Source: CAD feature listing. Evaluate the final solid. Frame: model axes, mm. Face numbers are marked on the shaded views. A direction names the side the tool comes from. Coordinates: 2 decimals unless noted, no trailing zeros. Loops run counter-clockwise (first coordinate to the right, second up) from the corner with the lowest first, then second, coordinate; pieces in that order, holes last. Notation, with made-up numbers: (-6.75, -27.75) - (21.25, -27.75) arc R21 ccw to (21.25, 1.25) - close; hole circle Ø9 at (64.5, 55). An arc over 180 degrees is marked (long way). Use CSV: the item, a comma, the result in double quotes. Start each with the question number.
```python
from build123d import *

# Parameters (mm, degrees)
BOSS_EXTRUDE1_DEPTH      = 28.22702
BOSS_EXTRUDE1_DEPTH_BACK = 27.08402
SKETCH2_R                = 40.9575
CUT_EXTRUDE1_DEPTH       = 152.701320166
CUT_EXTRUDE2_DEPTH       = 152.701320166


with BuildPart() as part:
    # Sketch1 → Boss-Extrude1 (new, two sides: drawn at the far end of the back side and taken through both)
    with BuildSketch(Plane(origin=(0, 0, 0), x_dir=(1, 0, 0), z_dir=(0, 1, 0)).offset(-BOSS_EXTRUDE1_DEPTH_BACK)):
        with BuildLine():
            Line((-35.721676258, -109.931199839), (-58.1025, -56.069211009))
            Line((-58.1025, -56.069211009), (-58.1025, -54.569599156))
            Line((-58.1025, -54.569599156), (-58.1025, 64.002262273))
            Line((-58.1025, 64.002262273), (-46.861446545, 91.314524953))
            ThreePointArc((-46.861446545, 91.314524953), (-41.24957855, 98.176226775), (-32.76841286, 100.75418))
            Line((-32.76841286, 100.75418), (30.359183597, 100.75418))
            ThreePointArc((30.359183597, 100.75418), (40.293026824, 97.071703902), (45.426195478, 87.803885872))
            Line((45.426195478, 87.803885872), (49.528165732, 60.811582924))
            ThreePointArc((49.528165732, 60.811582924), (51.439588659, 56.249062009), (55.27903878, 53.129966389))
            Line((55.27903878, 53.129966389), (78.152801145, 42.463755827))
            ThreePointArc((78.152801145, 42.463755827), (80.557519892, 40.354874086), (81.452537779, 37.284206824))
            Line((81.452537779, 37.284206824), (81.452537779, 31.863274858))
            ThreePointArc((81.452537779, 31.863274858), (80.517086587, 28.730043586), (78.016968856, 26.622528826))
            Line((78.016968856, 26.622528826), (63.334487079, 20.236471377))
            ThreePointArc((63.334487079, 20.236471377), (58.494345864, 15.83382392), (57.342134405, 9.393118961))
            Line((57.342134405, 9.393118961), (57.442982796, 8.729503635))
            ThreePointArc((57.442982796, 8.729503635), (57.930235286, 4.470832805), (58.1021964, 0.187828999))
            ThreePointArc((58.1021964, 0.187828999), (59.236377824, -4.444212154), (62.359072928, -8.048507927))
            Line((62.359072928, -8.048507927), (79.05801487, -19.969280438))
            ThreePointArc((79.05801487, -19.969280438), (80.818765563, -22.004906493), (81.452537779, -24.620694942))
            Line((81.452537779, -24.620694942), (81.452537779, -33.663524119))
            ThreePointArc((81.452537779, -33.663524119), (80.557519892, -36.73419138), (78.152801145, -38.843073121))
            Line((78.152801145, -38.843073121), (63.968698461, -45.457228827))
            ThreePointArc((63.968698461, -45.457228827), (59.714275337, -49.174099767), (58.102788562, -54.588742513))
            ThreePointArc((58.102788562, -54.588742513), (58.102572141, -54.627028957), (58.1025, -54.665315944))
            Line((58.1025, -54.665315944), (58.1025, -56.069211009))
            Line((58.1025, -56.069211009), (35.721676258, -109.931199839))
            ThreePointArc((35.721676258, -109.931199839), (32.447083012, -113.91449974), (27.512189111, -115.40998))
            Line((27.512189111, -115.40998), (-27.512189111, -115.40998))
            ThreePointArc((-27.512189111, -115.40998), (-32.447083012, -113.91449974), (-35.721676258, -109.931199839))
        make_face()
    extrude(amount=BOSS_EXTRUDE1_DEPTH + BOSS_EXTRUDE1_DEPTH_BACK)

    # Sketch2 → Cut-Extrude1 (cut, through all)
    with BuildSketch(Plane(origin=(0, 28.22702, 0), x_dir=(1, 0, 0), z_dir=(0, 1, 0))):
        with Locations(Location((0, 0, 0), (0, 0, 270))):
            Circle(SKETCH2_R)
    extrude(amount=-CUT_EXTRUDE1_DEPTH, mode=Mode.SUBTRACT)

    # Sketch3 → Cut-Extrude2 (cut, through all)
    with BuildSketch(Plane(origin=(0, 28.22702, 0), x_dir=(1, 0, 0), z_dir=(0, 1, 0))):
        with BuildLine():
            Line((25.4, 86.078568), (-25.4, 86.078568))
            ThreePointArc((-25.4, 86.078568), (-33.081115057, 79.561637348), (-27.902461028, 70.921529936))
            ThreePointArc((-27.902461028, 70.921529936), (-26.668169348, 70.612352943), (-25.4, 70.508368))
            Line((-25.4, 70.508368), (25.4, 70.508368))
            ThreePointArc((25.4, 70.508368), (26.668169348, 70.612352943), (27.902461028, 70.921529936))
            ThreePointArc((27.902461028, 70.921529936), (33.081115057, 79.561637348), (25.4, 86.078568))
        make_face()
    extrude(amount=-CUT_EXTRUDE2_DEPTH, mode=Mode.SUBTRACT)


solid = part.part
```
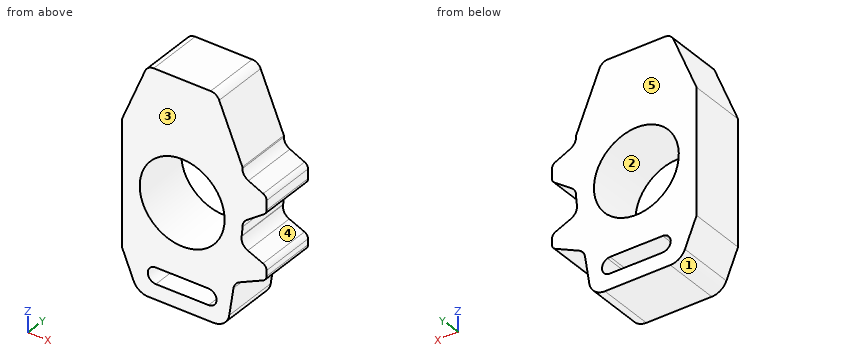
(1) Pin query (flat end, axial travel): pin 1 Ø1 at (y, z) = (-18.5, -73) entering from -X; pin 2 Ø1 at (y, z) = (15.5, -48) entering from +X. Return the tip coordinate at first contact, or that it passes through.
(2) Draft query along X for the marked faces 1, 2 and 3. Return one class per face: released by +X, released by -X, zero draft, split by the parting line, or undercut.
(3) Ray query, line 1 (Z direction, x = -20, y = 4); line 2 (X direction, y = 10, z = 0); line 3 (Z direction, x = -20.5, y = 23.5). Return the intervals inside material, ascending. Write a range as [from, to].
(4) Reachability of the marked faces 4 and 5 from +Z, -Z, +X, -X, +Y, -Y: full face, straight path, thin tool, end or side. Return the list, or none.
(5) Section B-B on y = 1. State how many separate pieces and enclosed holes the cut face has, plus the area to 3 significant figures.
(6) Section A-A on x = 0. Output: boundary loops of the cut face in (y, z), plus the area to 3 significant figures.
(7) Section C-C on z = -46. Output: boundary loops of the cut face in (x, y), plus the area to 3 significant figures.
Solution:
1,pin 1,"stops at x = -54.61"
1,pin 2,"stops at x = 67.35"
2,face 1,"released by -X"
2,face 2,"undercut"
2,face 3,"zero draft"
3,line 1,"z = [-100.75, -86.08], [-70.51, -35.74], [35.74, 115.41]"
3,line 2,"x = [-58.1, -40.96], [40.96, 58.1]"
3,line 3,"z = [-100.75, -86.08], [-70.51, -35.46], [35.46, 115.41]"
4,face 4,"+X, +Y, -Y"
4,face 5,"+Z, -Z, +X, -X, +Y"
5,separate pieces,"1"
5,enclosed holes,"2"
5,area,"17,800 mm²"
6,outline,"(-27.08, -100.75) - (28.23, -100.75) - (28.23, -86.08) - (-27.08, -86.08) - close; (-27.08, -70.51) - (28.23, -70.51) - (28.23, -40.96) - (-27.08, -40.96) - close; (-27.08, 40.96) - (28.23, 40.96) - (28.23, 115.41) - (-27.08, 115.41) - close"
6,area,"6,560 mm²"
7,outline,"(-58.1, -27.08) - (70.57, -27.08) - (70.57, 28.23) - (-58.1, 28.23) - close"
7,area,"7,120 mm²"
